from build123d import *
from build123d.topology import SkipClean

# Parameters (mm, degrees)
ESQUISSE1_R        = 6.1
ESQUISSE1_R_2      = 1.5
BOSS_EXTRU_1_DEPTH = 1
BOSS_EXTRU_2_START = 10
ESQUISSE2_R        = 4.5
ESQUISSE2_R_2      = 1.5
BOSS_EXTRU_2_DEPTH = 10
BOSS_EXTRU_3_START = 1
ESQUISSE3_R        = 6.1
ESQUISSE3_R_2      = 1.5
BOSS_EXTRU_3_DEPTH = 1


with BuildPart() as part:
    # Esquisse1 → Boss.-Extru.1 (new body)
    with BuildSketch(Plane.XY):
        Circle(ESQUISSE1_R)
        Circle(ESQUISSE1_R_2, mode=Mode.SUBTRACT)
    extrude(amount=BOSS_EXTRU_1_DEPTH)

    # Esquisse2 → Boss.-Extru.2 (add)
    with SkipClean():  # the faces are left unmerged after this step: merging them gives an invalid solid
        with BuildSketch(Plane(origin=(0, 0, 0), x_dir=(-1, 0, 0), z_dir=(0, 0, -1)).offset(BOSS_EXTRU_2_START)):
            Circle(ESQUISSE2_R)
            Circle(ESQUISSE2_R_2, mode=Mode.SUBTRACT)
        extrude(amount=-BOSS_EXTRU_2_DEPTH)

    # Esquisse3 → Boss.-Extru.3 (add)
    with SkipClean():  # the faces are left unmerged after this step: merging them gives an invalid solid
        with BuildSketch(Plane(origin=(0, 0, -10), x_dir=(-1, 0, 0), z_dir=(0, 0, -1)).offset(BOSS_EXTRU_3_START)):
            with Locations(Location((0, 0, 0), (0, 0, 180))):
                Circle(ESQUISSE3_R)
            Circle(ESQUISSE3_R_2, mode=Mode.SUBTRACT)
        extrude(amount=-BOSS_EXTRU_3_DEPTH)


solid = part.part
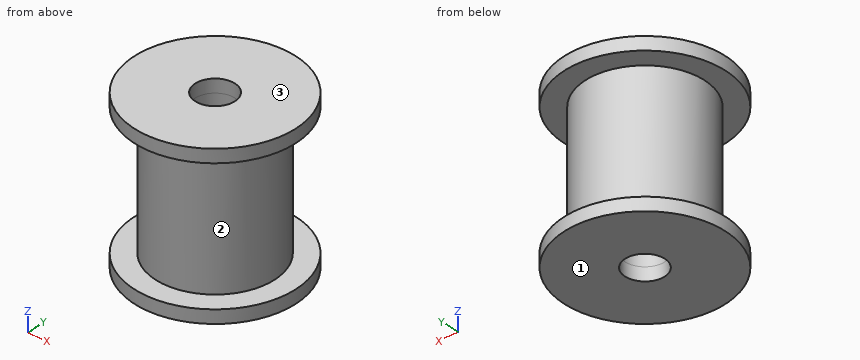
Could you check a few things on this model? Use its own coordinates, in mm. Face numbers are marked on the shaded views. Coordinates: 2 decimals unless noted, no trailing zeros. Write each loop counter-clockwise with the first axis right and the second up, starting at its lowest first coordinate (ties: lowest second). Pieces come first, ordered by that corner, then holes. Notation, with made-up numbers: (-7, -14) - (6, -14) arc R10 ccw to (6, 4) - close; hole circle Ø7 at (-29.5, 89). An arc over 180 degrees is marked (long way). Write item = value, one per line.
1) Suppose I cut it at C-C on z = -6.5. Please give me the cut outline in (x, y).
Result set:
outline = circle Ø9 at (0, 0); hole circle Ø3 at (0, 0)
2) Suppose I cut it at D-D on x = -1.75. Please give me the cut outline in (y, z), plus the area to 3 significant figures.
Result set:
outline = (-5.84, -11) - (5.84, -11) - (5.84, -10) - (4.15, -10) - (4.15, 0) - (5.84, 0) - (5.84, 1) - (-5.84, 1) - (-5.84, 0) - (-4.15, 0) - (-4.15, -10) - (-5.84, -10) - close
area = 106 mm2
3) Will these pins go through, and if not, where does the flat tip stop? pin 1 Ø1 at (x, z) = (-2.5, -1.5) entering from +Y; pin 2 Ø2.5 at (x, y) = (0, 0) entering from -Z; pin 3 Ø2 at (y, z) = (3.5, -4) entering from +X; pin 4 Ø3 at (y, z) = (4.5, -2.5) entering from -X.
Result set:
pin_1 = 4.03
pin_2 = through
pin_3 = 3.74
pin_4 = -3.35
4) We'd pull the mould along Z, two halves only. Please class the marked faces 1, 2 and 3: +Z half, -Z half, draft (parallel to the pull), parting line (faces both ways), or undercut.
Result set:
face_1 = -Z half
face_2 = undercut
face_3 = +Z half
5) Please list where these lines run through material, in increasing order: line 1 (Z direction, x = 5, y = -1.75); line 2 (Y direction, x = 0, z = -10.4); line 3 (Y direction, x = -0.5, z = -5.5). Write a range as [from, to].
Result set:
line_1 = [-11, -10], [0, 1]
line_2 = [-6.1, -1.5], [1.5, 6.1]
line_3 = [-4.47, -1.41], [1.41, 4.47]
6) Suppose I cut it at A-A on y = 0. Please give me the cut outline in (x, z), plus the area to 3 significant figures.
Result set:
outline = (-6.1, -11) - (-1.5, -11) - (-1.5, 1) - (-6.1, 1) - (-6.1, 0) - (-4.5, 0) - (-4.5, -10) - (-6.1, -10) - close; (1.5, -11) - (6.1, -11) - (6.1, -10) - (4.5, -10) - (4.5, 0) - (6.1, 0) - (6.1, 1) - (1.5, 1) - close
area = 78.4 mm2
